```python
from build123d import *

# Parameters (mm, degrees)
STOCK_BASE_SKEWED_1_START     = 6.9
STOCK_BASE_SKEWED_1_OUTLINE_R = 1.2
STOCK_BASE_SKEWED_1_DEPTH     = 1.1
SKETCH1_W                     = 2.5
SKETCH1_H                     = 1.5
BOSS_EXTRUDE1_DEPTH           = 8.991987159


# Read off the part's stored shape, not the designer's step: Stock-Base_skewed-1
with BuildPart() as part:
    # Stock-Base_skewed-1 outline → Stock-Base_skewed-1 (new body)
    with BuildSketch(Plane.XY.offset(STOCK_BASE_SKEWED_1_START)):
        with BuildLine():
            ThreePointArc((8.999971655, 10.488095238), (7.184905048, 12.904351279), (4.369026688, 11.807269193))
            Line((4.369026688, 11.807269193), (-2.088353846, 1.281123809))
            ThreePointArc((-2.088353846, 1.281123809), (-2.417250501, -0.399249317), (-1.565479113, -1.884615385))
            ThreePointArc((-1.565479113, -1.884615385), (-1.415835135, -1.970269972), (-1.245993579, -2))
            Line((-1.245993579, -2), (-1.245993579, -7))
            Line((-1.245993579, -7), (7.745993579, -7))
            Line((7.745993579, -7), (7.745993579, -2))
            ThreePointArc((7.745993579, -2), (7.915835135, -1.970269972), (8.065479113, -1.884615385))
            ThreePointArc((8.065479113, -1.884615385), (8.715388585, -1.046209071), (8.949972222, -0.011666667))
            Line((8.949972222, -0.011666667), (8.999971655, 10.488095238))
        make_face()
        Circle(STOCK_BASE_SKEWED_1_OUTLINE_R, mode=Mode.SUBTRACT)
        with Locations((6.5, 0)):
            Circle(STOCK_BASE_SKEWED_1_OUTLINE_R, mode=Mode.SUBTRACT)
        with BuildLine():
            Line((0.632085047, 2.847123137), (4.449478669, 9.069838376))
            ThreePointArc((4.449478669, 9.069838376), (5.815094952, 8.095648721), (7.489077768, 8.203976226))
            Line((7.489077768, 8.203976226), (7.463119607, 2.75282442))
            ThreePointArc((7.463119607, 2.75282442), (7.325518036, 2.467571215), (7.017292273, 2.394766941))
            ThreePointArc((7.017292273, 2.394766941), (4.297058288, 1.072169676), (4.934520887, -1.884615385))
            ThreePointArc((4.934520887, -1.884615385), (5.084164865, -1.970269972), (5.254006421, -2))
            Line((5.254006421, -2), (1.245993579, -2))
            ThreePointArc((1.245993579, -2), (1.415835135, -1.970269972), (1.565479113, -1.884615385))
            ThreePointArc((1.565479113, -1.884615385), (2.412392059, 0.427626653), (0.822306837, 2.307880297))
            ThreePointArc((0.822306837, 2.307880297), (0.598713954, 2.532178772), (0.632085047, 2.847123137))
        make_face(mode=Mode.SUBTRACT)
        with Locations((6.5, 10.5)):
            Circle(STOCK_BASE_SKEWED_1_OUTLINE_R, mode=Mode.SUBTRACT)
    extrude(amount=STOCK_BASE_SKEWED_1_DEPTH)

    # Sketch1 → Boss-Extrude1 (add)
    with BuildSketch(Plane(origin=(7.745993579, 0, 0), x_dir=(0, 0, -1), z_dir=(1, 0, 0))):
        with Locations((-9.25, -4.5)):
            Rectangle(SKETCH1_W, SKETCH1_H)
    extrude(amount=-BOSS_EXTRUDE1_DEPTH)


solid = part.part
```
Verification items for the finished model (mm, model axes). A direction names the side the tool comes from. Round coordinates to 2 decimals unless told otherwise and drop trailing zeros. Loops run counter-clockwise (first coordinate to the right, second up) from the corner with the lowest first, then second, coordinate; pieces in that order, holes last. Notation, with made-up numbers: (81, 62) -> (128, 62) arc R25 cw to (128, 86) -> close; hole circle Ø4 at (59.5, -11.75). An arc over 180 degrees is marked (long way). Answer as a JSON object with one key per item and string values.
Q1. Go/stop test with flat-tipped pins: P1, Ø2, axis at x = 6.5, y = 0, coming from the +Z side; P2, Ø2, axis at x = 3.5, z = 8.5, coming from the +Y side; P3, Ø0.8, axis at x = 2, z = 9.5, coming from the -Y side; P4, Ø2, axis at x = -0.5, y = 0, coming from the +Z side. Record where each tip stops, or that it passes through.
Data:
{"P1": "passes through", "P2": "stops at y = 11.8", "P3": "stops at y = -5.25", "P4": "stops at z = 8"}
Q2. Section check B-B (z = 7.65). Record the boundary of the cut face in (x, y).
Data:
{"outline": "(-2.09, 1.28) arc R2.45 ccw to (-1.57, -1.88) arc R0.5 ccw to (-1.25, -2) -> (-1.25, -7) -> (7.75, -7) -> (7.75, -2) arc R0.5 ccw to (8.07, -1.88) arc R2.45 ccw to (8.95, -0.01) -> (9, 10.49) arc R2.5 ccw to (4.37, 11.81) -> close; hole circle Ø2.4 at (0, 0); hole (0.63, 2.85) arc R0.37 ccw to (0.82, 2.31) arc R2.45 cw to (1.57, -1.88) arc R0.5 cw to (1.25, -2) -> (5.25, -2) arc R0.5 cw to (4.93, -1.88) arc R2.45 cw to (7.02, 2.39) arc R0.37 ccw to (7.46, 2.75) -> (7.49, 8.2) arc R2.5 cw to (4.45, 9.07) -> close; hole circle Ø2.4 at (6.5, 0); hole circle Ø2.4 at (6.5, 10.5)"}
Q3. Section check C-C (y = 7). Record the boundary of the cut face in (x, z).
Data:
{"outline": "(1.42, 6.9) -> (3.18, 6.9) -> (3.18, 8) -> (1.42, 8) -> close; (7.48, 6.9) -> (8.98, 6.9) -> (8.98, 8) -> (7.48, 8) -> close"}
Q4. Draft check along Y on faces 6 (the cylindrical face through (2.42, 0.39, 7.44)), 7 (the flat face through (3.2, -7, 7.4)), 8 (the flat face through (4.5, 1, 8)). Enter one of: pulls with the +Y half, pulls with the -Y half, needs draft (parallel to the pull), parting line crosses it, or undercut.
Data:
{"face 6": "undercut", "face 7": "pulls with the -Y half", "face 8": "needs draft"}
Q5. Section check D-D (x = -0.25). Record the boundary of the cut face in (y, z), then the cut area to 3 significant figures.
Data:
{"outline": "(-7, 6.9) -> (-1.17, 6.9) -> (-1.17, 8) -> (-3.75, 8) -> (-3.75, 10.5) -> (-5.25, 10.5) -> (-5.25, 8) -> (-7, 8) -> close; (1.17, 6.9) -> (4.28, 6.9) -> (4.28, 8) -> (1.17, 8) -> close", "area": "13.6 mm2"}
Q6. Access from +Z, -Z, +X, -X, +Y, -Y to the whole of each face (thin tool, end or side, straight path). Record for faces 1 (the flat face through (-1.246, -4, 8)), 2 (the flat face through (7.746, -5, 8)), 3 (the flat face through (3, -3.75, 9)), 4 (the flat face through (3, -5.25, 9)), 5 (the flat face through (2.51, 5.91, 7.44)).
Data:
{"face 1": "+Z, -Z, -X, -Y", "face 2": "+Z, -Z, +X, -Y", "face 3": "+Z, +X, -X, +Y", "face 4": "+Z, +X, -X, -Y", "face 5": "+Z, -Z"}
Q7. Section check A-A (x = 6.5). Record the boundary of the cut face in (y, z), then the cut area to 3 significant figures.
Data:
{"outline": "(-7, 6.9) -> (-1.2, 6.9) -> (-1.2, 8) -> (-3.75, 8) -> (-3.75, 10.5) -> (-5.25, 10.5) -> (-5.25, 8) -> (-7, 8) -> close; (1.2, 6.9) -> (2.45, 6.9) -> (2.45, 8) -> (1.2, 8) -> close; (8, 6.9) -> (9.3, 6.9) -> (9.3, 8) -> (8, 8) -> close; (11.7, 6.9) -> (13, 6.9) -> (13, 8) -> (11.7, 8) -> close", "area": "14.4 mm2"}
Q8. Scan lines: line 1 (Y direction, x = 6.5, z = 7.25); line 2 (Y direction, x = 4.75, z = 7.95); line 3 (Y direction, x = 5.5, z = 9.9). Record each from-to range of solid material in increasing order. Write a range as from..to.
Data:
{"line 1": "y = -7..-1.2, 1.2..2.45, 8..9.3, 11.7..13", "line 2": "y = -7..-2, -1.71..1.71, 8.71..12.29", "line 3": "y = -5.25..-3.75"}
